Autodesk Inventor part; units mm, degrees
ref_plane "YZ Plane" through (0, 0, 0) normal (1, 0, 0) x (0, 1, 0)
ref_plane "XZ Plane" through (0, 0, 0) normal (0, 1, 0) x (-1, 0, 0)
ref_plane "XY Plane" through (0, 0, 0) normal (0, 0, 1) x (1, 0, 0)
sketch "Sketch1" plane through (0, 0, 0) normal (0, 1, 0) x (-1, 0, 0)
  line L0 (0, 0) -> (812.8, 0)
  line L1 (812.8, 0) -> (812.8, -584.2)
  line L2 (812.8, -584.2) -> (0, -584.2)
  line L3 (0, -584.2) -> (0, 0)
  line L4 (-82.55, 82.55) -> (895.35, 82.55)
  line L5 (895.35, 82.55) -> (895.35, -666.75)
  line L6 (895.35, -666.75) -> (-82.55, -666.75)
  line L7 (-82.55, -666.75) -> (-82.55, 82.55)
  dimension "d0" = 812.8
  dimension "d1" = 584.2
  dimension "d2" = 82.55
  dimension "d3" = 82.55
  dimension "d4" = 82.55
  dimension "d5" = 82.55
extrude "Extrusion1" add sketch "Sketch1" along normal blind 127
fillet "Fillet1" radius 31.75 8 edges at (-406.4, 127, 82.55) (82.55, 127, -292.1) (-406.4, 0, 82.55) (82.55, 0, -292.1) (-895.35, 127, -292.1) (-406.4, 127, -666.75) (-406.4, 0, -666.75) (-895.35, 0, -292.1)
fillet "Fillet2" radius 31.75 12 edges at (-886.0506, 117.7006, 73.2506) (-886.0506, 9.2994, 73.2506) (-895.35, 63.5, 82.55) (-886.0506, 117.7006, -657.4506) (-886.0506, 9.2994, -657.4506) (-895.35, 63.5, -666.75) (73.2506, 117.7006, 73.2506) (73.2506, 9.2994, 73.2506) (82.55, 63.5, 82.55) (73.2506, 117.7006, -657.4506) (73.2506, 9.2994, -657.4506) (82.55, 63.5, -666.75)
properties part number "bumpers"
Could you check a few things on this model? Use its own coordinates, in mm. A direction names the side the tool comes from. Give positions to 0.01 mm unless a question says otherwise; leave off trailing zeros. Order: outer loops, then holes, each group sorted by start corner. A loop starts at its lowest first (then second) coordinate and runs counter-clockwise, first axis right, second up. Notation, with made-up numbers: (-38, 2.5) - (16, 2.5) arc R24 cw to (16, 22.5) - close; hole circle Ø8 at (62, -37). An arc over 180 degrees is marked (long way). Return JSON: item names as keys, results as strings. Group by question number.
Q1. Suppose I cut it at B-B, the plane x = -88. Please give me the cut outline in (y, z), and give its area (3 significant figures).
Q2. Please list where these lines run through material, in increasing order: line 1 along Z through (x, y) = (-268.5, 50.5); line 2 along X through (y, z) = (54.5, -284); line 3 along X through (y, z) = (98, -522.5). Write a range as [from, to].
Q3. Thinking about a two-plate mould opening in Z: for faces 3 (the face through (-895.35, 63, -287)), 4 (the face through (0, 63, -296)), 5 (the face through (-412.8, 9.05, 73)), which applies, pulls with the +Z half, pulls with the -Z half, needs draft (parallel to the pull), parting line crosses it, or undercut?
Q4. Will these pins go through, and if not, where does the flat tip stop? pin 1 Ø1 at (x, y) = (-614.5, 104.5) entering from -Z; pin 2 Ø10 at (x, y) = (-715, 17.5) entering from +Z.
Q5. Suppose I cut it at C-C, the plane y = 113.5. Please give me the cut outline in (x, z).
Q6. Suppose I cut it at A-A, the plane z = -289. Please give me the cut outline in (x, y).
Q7. Which directions (+Z, -Z, +X, -X, +Y, -Y) give clear straight access to the entire face, cutting with the end or side of a thin tool? Please do faces 1 (the face through (-413, 63, -666.75)), 2 (the face through (-812.8, 63, -288)).
Resolved:
{
 "1": {"outline": "(0, -635) arc R31.75 ccw to (31.75, -666.75) - (95.25, -666.75) arc R31.75 ccw to (127, -635) - (127, -584.2) - (0, -584.2) - close; (0, 0) - (127, 0) - (127, 50.8) arc R31.75 ccw to (95.25, 82.55) - (31.75, 82.55) arc R31.75 ccw to (0, 50.8) - close", "area": "20,100 mm2"},
 "2": {"line 1": "z = [-666.75, -584.2], [0, 82.55]", "line 2": "x = [-895.35, -812.8], [0, 82.55]", "line 3": "x = [-895.23, -812.8], [0, 82.43]"},
 "3": {"face 3": "needs draft", "face 4": "undercut", "face 5": "pulls with the +Z half"},
 "4": {"pin 1": "stops at z = -665.52", "pin 2": "stops at z = 81.17"},
 "5": {"outline": "(-889.58, -635) arc R25.98 ccw to (-863.6, -660.98) - (50.8, -660.98) arc R25.98 ccw to (76.78, -635) - (76.78, 50.8) arc R25.98 ccw to (50.8, 76.78) - (-863.6, 76.78) arc R25.98 ccw to (-889.58, 50.8) - close; hole (-812.8, -584.2) - (0, -584.2) - (0, 0) - (-812.8, 0) - close"},
 "6": {"outline": "(-895.35, 31.75) arc R31.75 ccw to (-863.6, 0) - (-812.8, 0) - (-812.8, 127) - (-863.6, 127) arc R31.75 ccw to (-895.35, 95.25) - close; (0, 0) - (50.8, 0) arc R31.75 ccw to (82.55, 31.75) - (82.55, 95.25) arc R31.75 ccw to (50.8, 127) - (0, 127) - close"},
 "7": {"face 1": "-Z, +X, -X, +Y, -Y", "face 2": "+Y, -Y"}
}
